```python
from build123d import *

# Parameters (mm, degrees)
F1_DEPTH  = 60
F2_T      = -1.5
F4_DEPTH  = 1.7
F6_DEPTH  = 1.5
F8_DEPTH  = 7.7
F9_DEPTH  = 0.1
F10_DEPTH = 0.4
F11_DEPTH = 0.5
F13_R     = 0.9
F14_DEPTH = 25
F15_DEPTH = 63.1
F17_DEPTH = 1.8
F19_DEPTH = 1.69
F20_DEPTH = 1.6
F21_DEPTH = 2
F22_DEPTH = 2
F23_DEPTH = 2
F24_DEPTH = 2
F25_DEPTH = 0.5
F26_DEPTH = 0.5
F27_DEPTH = 25
F28_DEPTH = 0.5


with BuildPart() as f1:
    # F0 (on Right) → F1 (new body)
    with BuildSketch(Plane.YZ):
        Polygon((16.1535342058, -7.67995), (16.1535342058, 0), (-25.1004657942, 7.67995), (-25.1004657942, 0), align=None)
    extrude(amount=F1_DEPTH)

    # F2
    f2_openings = [f1.faces().sort_by_distance(p)[0] for p in [
        (30, -4.473466, -3.839975),
    ]]
    offset(amount=F2_T, openings=f2_openings)

    # F3 (on face) → F4 (cut)
    with BuildSketch(Plane.XZ.offset(25.1004657942)):
        Polygon((30, 0), (37.3, 0), (58.5109069943, 0), (58.5109069943, 6.6873678006), (1.489095157, 6.6873678006), (1.489095157, 0), (22.7, 0), align=None)
    extrude(amount=-F4_DEPTH, mode=Mode.SUBTRACT)

    # F5 (on face) → F6 (cut)
    with BuildSketch(Plane(origin=(0, -0.8407565289, -4.5162494345), x_dir=(1, 0, 0), z_dir=(0, -0.1830181807, -0.9831095288))):
        Polygon((1.5, 23.1507361077), (58.5, 23.1507361077), (58.5109069943, 24.6765070987), (1.489095157, 24.6765070987), align=None)
    extrude(amount=-F6_DEPTH, mode=Mode.SUBTRACT)

    # F7 (on face) → F8 (join)
    with BuildSketch(Plane(origin=(0, 0, 6.6873678006), x_dir=(1, 0, 0), z_dir=(0, 0, -1))):
        Polygon((22.8000010757, 23.4004657942), (30.0000010757, 23.4004657942), (37.2000010757, 23.4004657942), (37.2000010757, 25.1004657942), (22.8000010757, 25.1004657942), align=None)
    extrude(amount=F8_DEPTH)

    # F9 (add): a face of the model
    f9_faces = [f1.faces().sort_by_distance(p)[0] for p in [
        (29.9999984717, -25.1004657942, 4.2501617501),
    ]]
    extrude(f9_faces, amount=F9_DEPTH)

    # F10 (add): a face of the model
    f10_faces = [f1.faces().sort_by_distance(p)[0] for p in [
        (29.9999984717, -25.2004657942, 4.2501617501),
    ]]
    extrude(f10_faces, amount=F10_DEPTH)

    # F11 (add): a face of the model
    f11_faces = [f1.faces().sort_by_distance(p)[0] for p in [
        (30.0000010757, -23.4004657942, 2.4125352339),
    ]]
    extrude(f11_faces, amount=F11_DEPTH)

    # F13 (on face) → F14 (join)
    with BuildSketch(Plane(origin=(22.8000010757, 0, 0), x_dir=(0, -1, 0), z_dir=(-1, 0, 0))):
        with Locations((24.2503285408, 2.1311247256)):
            Circle(F13_R)
    extrude(amount=F14_DEPTH)

    # F15 (cut): a face of the model
    f15_faces = [f1.faces().sort_by_distance(p)[0] for p in [
        (-2.1999989243, -24.2503285408, 2.1311247256),
    ]]
    extrude(f15_faces, amount=-F15_DEPTH, mode=Mode.SUBTRACT)

    # F16 (on face) → F17 (cut)
    with BuildSketch(Plane(origin=(0, 0, 0), x_dir=(0, -1, 0), z_dir=(-1, 0, 0))):
        Polygon((25.1004657942, 7.67995), (22.7930747999, -0.4295498004), (25.6004657942, 0), (25.6004657942, 7.67995), align=None)
    extrude(amount=-F17_DEPTH, mode=Mode.SUBTRACT)

    # F18 (on face) → F19 (cut)
    with BuildSketch(Plane.YZ.offset(60)):
        Polygon((-22.6419516364, -0.4576832745), (-25.1004657942, 7.67995), (-25.6004657942, 7.67995), (-25.6004657942, 0), align=None)
    extrude(amount=-F19_DEPTH, mode=Mode.SUBTRACT)

    # F20 (cut): a face of the model
    f20_faces = [f1.faces().sort_by_distance(p)[0] for p in [
        (30.0000010757, -24.2504657942, -1.0126321994),
    ]]
    extrude(f20_faces, amount=-F20_DEPTH, mode=Mode.SUBTRACT)

    # F21 (add): a face of the model
    f21_faces = [f1.faces().sort_by_distance(p)[0] for p in [
        (0, -3.8923715411, -0.0707367211),
    ]]
    extrude(f21_faces, amount=F21_DEPTH)

    # F22 (cut): faces of the model
    f22_faces = [f1.faces().sort_by_distance(p)[0] for p in [
        (1.5, -4.3223600686, -0.7846449221),
        (1.489095157, -23.887211668, 5.1322390537),
    ]]
    extrude(f22_faces, amount=-F22_DEPTH, mode=Mode.SUBTRACT)

    # F23 (add): a face of the model
    f23_faces = [f1.faces().sort_by_distance(p)[0] for p in [
        (60, -3.8610992798, -0.074441199),
    ]]
    extrude(f23_faces, amount=F23_DEPTH)

    # F24 (cut): faces of the model
    f24_faces = [f1.faces().sort_by_distance(p)[0] for p in [
        (58.5109069943, -23.8729043508, 5.1821889961),
        (58.5, -4.2998130012, -0.7863611565),
    ]]
    extrude(f24_faces, amount=-F24_DEPTH, mode=Mode.SUBTRACT)

    # F25 (cut): a face of the model
    f25_faces = [f1.faces().sort_by_distance(p)[0] for p in [
        (30, 14.6535342058, -4.3236166646),
    ]]
    extrude(f25_faces, amount=-F25_DEPTH, mode=Mode.SUBTRACT)

    # F26 (cut): a face of the model
    f26_faces = [f1.faces().sort_by_distance(p)[0] for p in [
        (30, 15.1535342058, -4.3236166646),
    ]]
    extrude(f26_faces, amount=-F26_DEPTH, mode=Mode.SUBTRACT)

    # F27 (cut): a face of the model
    f27_faces = [f1.faces().sort_by_distance(p)[0] for p in [
        (30, 15.1535342058, -7.4007061691),
    ]]
    extrude(f27_faces, amount=-F27_DEPTH, mode=Mode.SUBTRACT)

    # F28 (add): a face of the model
    f28_faces = [f1.faces().sort_by_distance(p)[0] for p in [
        (30, 15.6535342058, -4.4166979416),
    ]]
    extrude(f28_faces, amount=F28_DEPTH)


solid = f1.part
```
The model under review builds one solid part; all positions refer to its coordinate system, in mm. A direction names the side the tool comes from. Coordinates: 2 decimals unless noted, no trailing zeros. Write each loop counter-clockwise with the first axis right and the second up, starting at its lowest first coordinate (ties: lowest second). Pieces come first, ordered by that corner, then holes.
1) Machinability: for faces 4 (the face through (-1.39, -23.11, 0.69)), 5 (the face through (60.5, -4, -1)), 6 (the face through (30, -22.9, 3)), which of the approach directions +Z, -Z, +X, -X, +Y, -Y give a long, thin tool a straight path to every point of the face, cutting with its end or side? Answer none if there is none.
2) To check wall thickness, follow probe 1 along X at (y, z) = (-11.5, -2); probe 2 along Y at (x, z) = (56.5, -5.25); probe 3 along Z at (x, y) = (42.5, -15). State the ranges of each line that lie inside material, in increasing order.
3) We need section D-D on z = -5. State the section outline as (x, y) points.
4) Clearance check with flat-ended pins moving along their axes: pin 1 Ø5 at (x, y) = (50, -20.5) entering from +Z; pin 2 Ø2 at (x, z) = (13.5, -5) entering from -Y; pin 3 Ø5 at (x, y) = (38, 1.5) entering from -Z. State where each tip first meets the part, or that it passes through.
5) We need section C-C on y = -20. State the section outline as (x, z) points, then the cut area to 3 significant figures.
6) We need section B-B on x = 57.5. State the section outline as (y, z) points, then the cut area to 3 significant figures.
7) The part is to be moulded in two halves that separate along X. For faces 1 (the face through (61.24, -23, 0.73)), 2 (the face through (11, -24, 6.687)), 3 (the face through (62, -4, 0)), say which applies: pulls with the +X half, pulls with the -X half, needs draft (parallel to the pull), parting line crosses it, or undercut.
Answer list:
1. face 4: -Z, -X, -Y
1. face 5: -Z, -Y
1. face 6: -Z
2. probe 1: x = -2 to -0.5, 60.5 to 62
2. probe 2: y = 15.15 to 16.15
2. probe 3: z = 4.27 to 5.8
3. outline: (-2, 1.76) - (-0.5, 1.76) - (-0.5, 15.15) - (60.5, 15.15) - (60.5, 1.76) - (62, 1.76) - (62, 16.15) - (-2, 16.15) - close
4. pin 1: stops at z = 7.29
4. pin 2: stops at y = 15.15
4. pin 3: stops at z = 0.74
5. outline: (-2, -0.95) - (-0.5, -0.95) - (-0.5, 5.2) - (60.5, 5.2) - (60.5, -0.95) - (62, -0.95) - (62, 6.73) - (-2, 6.73) - close
5. area: 116 mm2
6. outline: (-25.6, 6.69) - (-23.4, 6.69) - (-23.4, 5.84) - (14.65, -1.25) - (15.15, -1.25) - (15.15, -7.59) - (15.65, -7.59) - (16.15, -7.68) - (16.15, 0) - (-25.1, 7.68) - (-25.6, 7.68) - close
6. area: 68.4 mm2
7. face 1: needs draft
7. face 2: undercut
7. face 3: pulls with the +X half
